Design review of the part built by this model. Coordinates are the model's own, in mm. Face numbers are marked on the shaded views. A direction names the side the tool comes from. Coordinates: 2 decimals unless noted, no trailing zeros. Loops run counter-clockwise (first coordinate to the right, second up) from the corner with the lowest first, then second, coordinate; pieces in that order, holes last. Notation, with made-up numbers: M 7.5,38 L 43.5,38 A35 ccw 43.5,70 Z; hole C 50,-27.5 d2. An arc over 180 degrees is marked long. Answer as a JSON object with one key per item and string values. Group by question number.
1. To check wall thickness, follow probe 1 along X at (y, z) = (-0.85, 1.15); probe 2 along Z at (x, y) = (1.5, -0.05); probe 3 along X at (y, z) = (-0.3, -0.15). State the ranges of each line that lie inside material, in increasing order.
2. Insertion check: pin 1 (1 mm diameter, centred on y = -1.5, z = -1.5, fed in from +X). The pin has a flat end and moves straight along its axis. Give the tip position at first contact, or say it passes through.
3. Consider section C-C (x = 3.25). State the section outline as (y, z) points, then the cut area to 3 significant figures.
4. Consider section D-D (x = -1). State the section outline as (y, z) points, then the cut area to 3 significant figures.
5. Consider section A-A (z = 0). State the section outline as (x, y) points, then the cut area to 3 significant figures.
6. Machinability: for the marked faces 1 and 2, which of the approach directions +Z, -Z, +X, -X, +Y, -Y give a long, thin tool a straight path to every point of the face, cutting with its end or side? Answer none if there is none.
7. Consider section B-B (y = 0). State the section outline as (x, z) points, then the cut area to 3 significant figures.
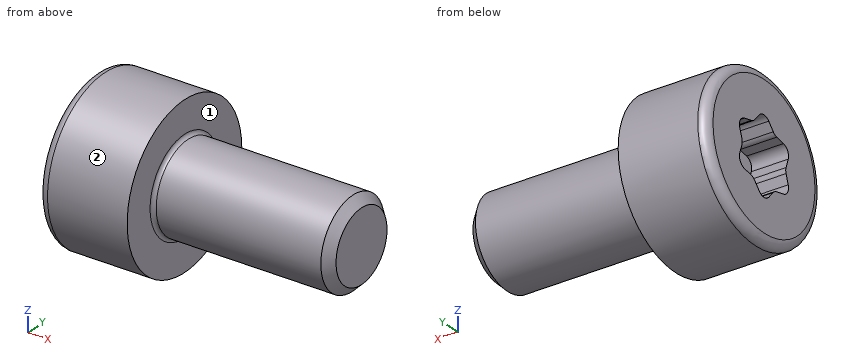
Autodesk Inventor part; units mm, degrees
ref_plane "YZ Plane" through (0, 0, 0) normal (1, 0, 0) x (0, 1, 0)
ref_plane "XZ Plane" through (0, 0, 0) normal (0, 1, 0) x (-1, 0, 0)
ref_plane "XY Plane" through (0, 0, 0) normal (0, 0, 1) x (1, 0, 0)
sketch "Sketch1" plane through (0, 0, 0) normal (0, 0, 1) x (1, 0, 0)
  line L0 (0, 0) -> (5, 0)
  line L1 (5, 0) -> (5, 1.25)
  line L2 (5, 1.25) -> (0, 1.25)
  line L3 (0, 1.25) -> (0, 0)
  line L4 (0, 0) -> (-2.5, 0)
  line L5 (-2.5, 0) -> (-2.5, 2.25)
  line L6 (-2.5, 2.25) -> (0, 2.25)
  line L7 (0, 2.25) -> (0, 0)
  dimension "d0" = 2.5
  dimension "d1" = 4.5
  dimension "d2" = 2.5
  dimension "d3" = 5
revolve "Revolution1" add sketch "Sketch1" angle 360 about axis through (0, 0, 0) along (1, 0, 0)
thread "Thread1"
sketch "Sketch2" plane through (-2.5, 0, 0) normal (-1, 0, 0) x (0, 0, 1)
  circle A0 centre (0, 0) radius 1.2 construction
  circle A1 centre (0, 0) radius 0.84 construction
  line L0 (-0.7275, -0.42) -> (-1.2, 0)
  line L1 (0, 0) -> (-0.7275, -0.42)
  line L2 (0, 0) -> (-0.7275, 0.42)
  line L3 (-3.15, 0) -> (3.15, 0) construction
  line L4 (-1.2, 0) -> (-0.7275, 0.42)
  dimension "d21" = 2.4
  dimension "d19" = 60
  dimension "d20" = 30
  dimension "d26" = 1.68
extrude "Extrusion1" cut sketch "Sketch2" against normal blind 1.04
pattern_circular "Circular Pattern1" count 6 over 360 about axis through (-2.5, 0, 0) along (1, 0, 0) of "Extrusion1"
fillet "Fillet2" radius 0.25 6 edges at (-1.98, 1.0392, -0.6) (-1.98, 1.0392, 0.6) (-1.98, 0, 1.2) (-1.98, -1.0392, 0.6) (-1.98, -1.0392, -0.6) (-1.98, 0, -1.2)
fillet "Fillet3" radius 0.25 6 edges at (-1.98, 0.84, 0) (-1.98, 0.42, -0.7275) (-1.98, -0.42, -0.7275) (-1.98, -0.84, 0) (-1.98, -0.42, 0.7275) (-1.98, 0.42, 0.7275)
fillet "Fillet4" radius 0.25 1 edges at (-2.5, -2.25, 0)
fillet "Fillet5" radius 0.1 1 edges at (0, -1.25, 0)
chamfer "Chamfer2" distance 0.25 angle 45 1 edges at (5, -1.25, 0)
equation "\"d0\" = d"
equation "\"d1\" = dk"
equation "\"d2\" = k"
equation "\"d3\" = l_"
equation "\"d6\" = b"
equation "\"d21\" = A_"
equation "\"d20\" = 0.5 * d19"
equation "\"d26\" = 0.7 * d21"
equation "\"d27\" = t"
equation "\"d32\" = v"
equation "\"d33\" = v"
equation "\"d34\" = v"
equation "\"d35\" = r"
equation "\"d36\" = v"
equation "\"A_\" = 2.4"
equation "\"d\" = 2.5"
equation "\"dk\" = 4.5"
equation "\"k\" = 2.5"
equation "\"l_\" = 5"
equation "\"lg\" = 0"
equation "\"t\" = 1.04"
equation "\"w\" = 0.55"
equation "\"v\" = 0.25"
equation "\"r\" = 0.1"
equation "\"da\" = 2.6"
equation "\"p\" = 0.45"
equation "\"ds_\" = d"
equation "\"GAL\" = 0.61345 * p"
equation "\"ls\" = 0"
equation "\"b\" = l_ - lg"
properties part number "Inbusschraube mit Innenrund ISO 14579 - M2,5x5-8.8" material "Stahl"
Findings below:
{
 "1": {"probe 1": "x = -2.5 to 0", "probe 2": "z = -1.25 to 1.25", "probe 3": "x = -1.46 to 5"},
 "2": {"pin 1": "stops at x = 0"},
 "3": {"outline": "C 0,0 d2.5", "area": "4.91 mm^2"},
 "4": {"outline": "C 0,0 d4.5", "area": "15.9 mm^2"},
 "5": {"outline": "M -2.5,-2 A0.25 ccw -2.25,-2.25 L 0,-2.25 L 0,-1.35 A0.1 cw 0.1,-1.25 L 4.75,-1.25 L 5,-1 L 5,1 L 4.75,1.25 L 0.1,1.25 A0.1 cw 0,1.35 L 0,2.25 L -2.25,2.25 A0.25 ccw -2.5,2 L -2.5,0.85 L -1.46,0.85 L -1.46,-0.85 L -2.5,-0.85 Z", "area": "21.9 mm^2"},
 "6": {"face 1": "+X", "face 2": "+X, -X"},
 "7": {"outline": "M -2.5,-2 A0.25 ccw -2.25,-2.25 L 0,-2.25 L 0,-1.35 A0.1 cw 0.1,-1.25 L 4.75,-1.25 L 5,-1 L 5,1 L 4.75,1.25 L 0.1,1.25 A0.1 cw 0,1.35 L 0,2.25 L -2.25,2.25 A0.25 ccw -2.5,2 L -2.5,1.07 L -1.46,1.07 L -1.46,-1.07 L -2.5,-1.07 Z", "area": "21.4 mm^2"}
}
